from build123d import *

# Parameters (mm, degrees)
SKETCH1_W                           = 76.2
SKETCH1_H                           = 76.2
BOSS_EXTRUDE1_DEPTH                 = 2.54
SKETCH2_W                           = 14.9
SKETCH2_H                           = 15.8
SKETCH2_W_2                         = 15.8
SKETCH2_H_2                         = 14.9
BOSS_EXTRUDE2_DEPTH                 = 7.1
F_9_64_0_14063_DIAMETER_HOLE1_D     = 3.572002
F_9_64_0_14063_DIAMETER_HOLE1_DEPTH = 5.7404
F_9_64_0_14063_DIAMETER_HOLE1_TIP   = 1.073137666


with BuildPart() as part:
    # Sketch1 → Boss-Extrude1 (new body)
    with BuildSketch(Plane(origin=(0, 0, 0), x_dir=(1, 0, 0), z_dir=(0, 1, 0))):
        Rectangle(SKETCH1_W, SKETCH1_H)
    extrude(amount=BOSS_EXTRUDE1_DEPTH)

    # Sketch2 → Boss-Extrude2 (add)
    with BuildSketch(Plane(origin=(0, 2.54, 0), x_dir=(1, 0, 0), z_dir=(0, 1, 0))):
        with Locations((-30.777, -21.31)):
            Rectangle(SKETCH2_W, SKETCH2_H)
        with Locations((-30.523, 21.31)):
            Rectangle(SKETCH2_W, SKETCH2_H)
        with Locations((-6.07, 30.523)):
            Rectangle(SKETCH2_W_2, SKETCH2_H_2)
        with Locations((17.7818, 30.523)):
            Rectangle(SKETCH2_W_2, SKETCH2_H_2)
        with Locations((30.523, 6.07)):
            Rectangle(SKETCH2_W, SKETCH2_H)
        with Locations((-30.523, -0.372526433)):
            Rectangle(SKETCH2_W, SKETCH2_H)
    extrude(amount=BOSS_EXTRUDE2_DEPTH)

    # 9/64 (0.14063) Diameter Hole1
    with Locations(Plane(origin=(0, 2.54, 0), x_dir=(1, 0, 0), z_dir=(0, 1, 0))):
        with Locations((34.29, -34.29), (-34.29, -34.29), (-34.29, 34.29), (34.29, 34.29)):
            Hole(F_9_64_0_14063_DIAMETER_HOLE1_D / 2, depth=F_9_64_0_14063_DIAMETER_HOLE1_DEPTH)
            with Locations((0, 0, -(F_9_64_0_14063_DIAMETER_HOLE1_DEPTH + F_9_64_0_14063_DIAMETER_HOLE1_TIP / 2))):  # 118° drill point
                Cone(0, F_9_64_0_14063_DIAMETER_HOLE1_D / 2, F_9_64_0_14063_DIAMETER_HOLE1_TIP, mode=Mode.SUBTRACT)


solid = part.part
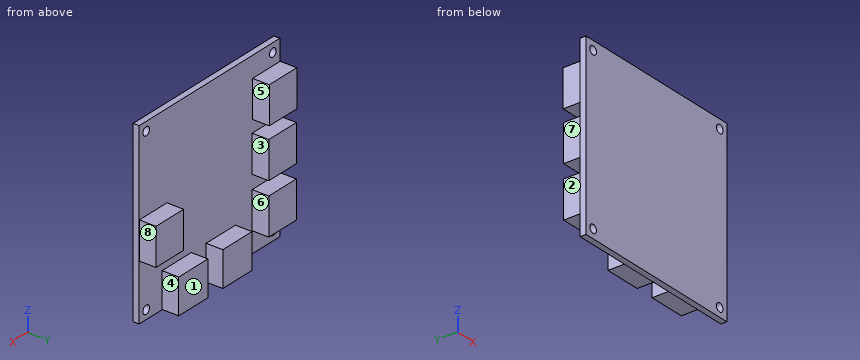
Check sheet for the modelled part. Datum: model origin and axes. Units: mm. Face numbers are marked on the shaded views. A direction names the side the tool comes from. Round coordinates to 2 decimals unless told otherwise and drop trailing zeros. Order: outer loops, then holes, each group sorted by start corner. A loop starts at its lowest first (then second) coordinate and runs counter-clockwise, first axis right, second up. Notation, with made-up numbers: M -11.5,86 L 26.5,86 A27 cw 26.5,109 Z; hole C -22,67.25 d3. An arc over 180 degrees is marked long. One line per item, written item: value. Start each with the question number.
1. Scan lines: line 1 along X through (y, z) = (1.6, -34.29); line 2 along Z through (x, y) = (-27, 4.75). Record each from-to range of solid material in increasing order.
2. Section check A-A on z = -34.29. Enter the section's corners in (x, y).
3. Section check C-C on x = 34.29. Enter the section's corners in (y, z).
4. Section check B-B on y = 3.75. Enter the section's corners in (x, z), and give its area (3 significant figures).
5. Access from +Z, -Z, +X, -X, +Y, -Y to the whole of each face (thin tool, end or side, straight path). Record for the marked faces 4, 5, 6, 7 and 8.
6. Release check for a two-part mould opening along X. For the marked faces 1, 2 and 3 record: released by +X, released by -X, zero draft, split by the parting line, or undercut.
7. Section check D-D on z = 6. Enter the section's corners in (x, y).
8. Gauge pin test, flat ends, axial feed: P1, Ø3, axis at x = -4, y = 7, coming from the +Z side; P2, Ø5, axis at x = 26.5, y = 7.5, coming from the -Z side; P3, Ø2, axis at x = -30, y = 6, coming from the -Z side. Record the tip position at first contact, or that the pin passes through.
Results found:
1. line 1: -38.1 to -36.08, -32.5 to 32.5, 36.08 to 38.1
1. line 2: -29.21 to -13.41, -7.53 to 8.27, 13.41 to 29.21
2. outline: M -38.1,0 L -36.08,0 L -36.08,2.54 L -38.1,2.54 Z; M -32.5,0 L 32.5,0 L 32.5,2.54 L 25.68,2.54 L 25.68,9.64 L 9.88,9.64 L 9.88,2.54 L 1.83,2.54 L 1.83,9.64 L -13.97,9.64 L -13.97,2.54 L -32.5,2.54 Z; M 36.08,0 L 38.1,0 L 38.1,2.54 L 36.08,2.54 Z
3. outline: M 0,-38.1 L 2.54,-38.1 L 2.54,-36.08 L 0,-36.08 Z; M 0,-32.5 L 2.54,-32.5 L 2.54,-13.97 L 9.64,-13.97 L 9.64,1.83 L 2.54,1.83 L 2.54,32.5 L 0,32.5 Z; M 0,36.08 L 2.54,36.08 L 2.54,38.1 L 0,38.1 Z
4. outline: M -38.23,13.41 L -23.33,13.41 L -23.33,29.21 L -38.23,29.21 Z; M -37.97,-29.21 L -23.07,-29.21 L -23.07,-13.41 L -37.97,-13.41 Z; M -37.97,-7.53 L -23.07,-7.53 L -23.07,8.27 L -37.97,8.27 Z; M -13.97,-37.97 L 1.83,-37.97 L 1.83,-23.07 L -13.97,-23.07 Z; M 9.88,-37.97 L 25.68,-37.97 L 25.68,-23.07 L 9.88,-23.07 Z; M 23.07,-13.97 L 37.97,-13.97 L 37.97,1.83 L 23.07,1.83 Z
4. area: 1,410 mm^2
5. face 4: -Z, +X, +Y
5. face 5: +Z, +X, +Y
5. face 6: +Z, -Z, +Y
5. face 7: -Z, -X, +Y
5. face 8: +Z, -Z, +X, +Y
6. face 1: zero draft
6. face 2: released by -X
6. face 3: undercut
7. outline: M -38.1,0 L 38.1,0 L 38.1,2.54 L -23.07,2.54 L -23.07,9.64 L -37.97,9.64 L -37.97,2.54 L -38.1,2.54 Z
8. P1: z = -23.07
8. P2: z = -37.97
8. P3: z = -29.21
